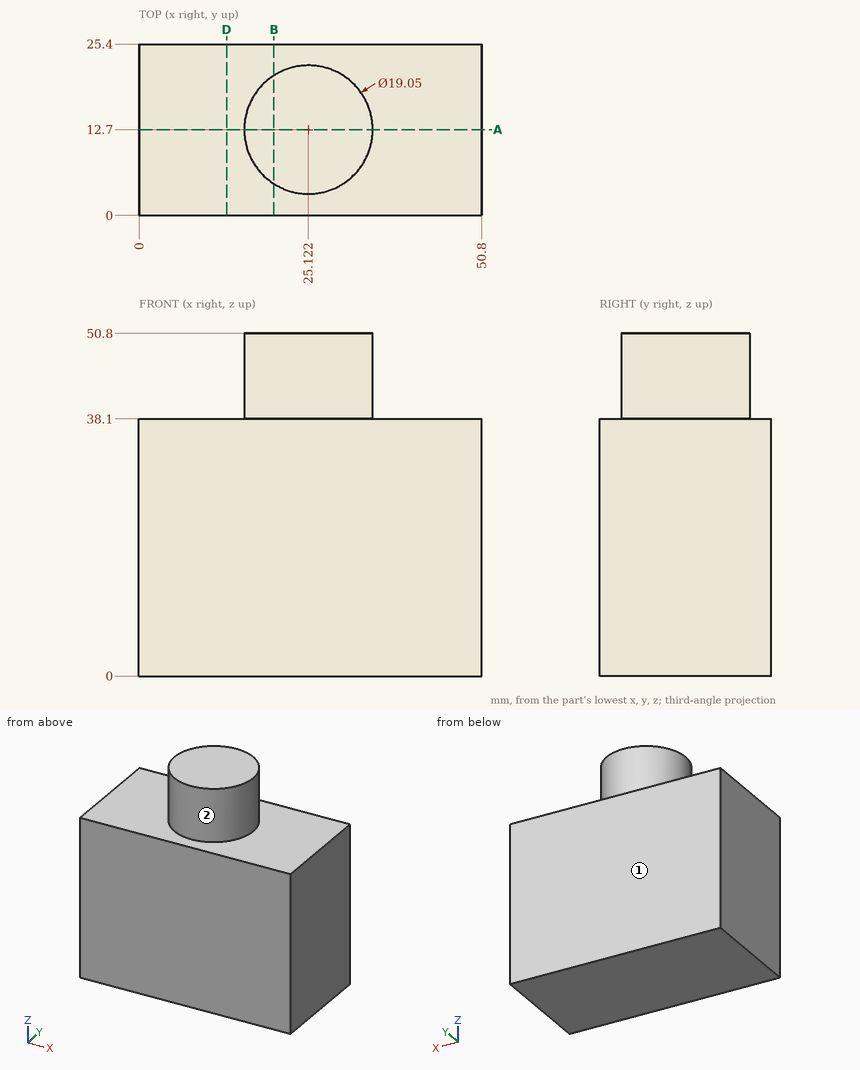
Geometry check sheet. Reference: drawing and pictorial views, mm from the part's lowest x, y, z. A direction names the side the tool comes from. Round coordinates to 2 decimals unless told otherwise and drop trailing zeros. Order: outer loops, then holes, each group sorted by start corner. A loop starts at its lowest first (then second) coordinate and runs counter-clockwise, first axis right, second up.
Q1. Cross-section at A-A, the plane y = 12.7. Enter the section's corners in (x, z), plus the area to 3 significant figures.
Filled sheet:
outline: (0, 0) - (50.8, 0) - (50.8, 38.1) - (34.65, 38.1) - (34.65, 50.8) - (15.6, 50.8) - (15.6, 38.1) - (0, 38.1) - close
area: 2,180 mm2
Q2. Scan lines: L1, parallel to Z at x = 20, y = 22.75; L2, parallel to X at y = 13.25, z = 47; L3, parallel to X at y = 16, z = 43.5. Record each from-to range of solid material in increasing order.
Filled sheet:
L1: z = 0 to 38.1
L2: x = 15.61 to 34.63
L3: x = 16.19 to 34.06
Q3. Depth check by flat-ended pin: P1, Ø5, axis at x = 33.5, z = 42.5, coming from the -Y side (1 decimal); P2, Ø10, axis at x = 41, y = 3.5, coming from the +Z side; P3, Ø6, axis at y = 6, z = 44, coming from the -X side (1 decimal). Enter the tip coordinate at first touch or a pass-through.
Filled sheet:
P1: stops at y = 5.2
P2: stops at z = 38.1
P3: stops at x = 16.3
Q4. Cross-section at D-D, the plane x = 13. Enter the section's corners in (y, z), plus the area to 3 significant figures.
Filled sheet:
outline: (0, 0) - (25.4, 0) - (25.4, 38.1) - (0, 38.1) - close
area: 968 mm2
Q5. Cross-section at B-B, the plane x = 20. Enter the section's corners in (y, z).
Filled sheet:
outline: (0, 0) - (25.4, 0) - (25.4, 38.1) - (20.73, 38.1) - (20.73, 50.8) - (4.67, 50.8) - (4.67, 38.1) - (0, 38.1) - close
Q6. Set-up check for the marked faces 1 and 2: record each of +Z, -Z, +X, -X, +Y, -Y from which the full face is reachable in a straight line by a thin tool's end or side.
Filled sheet:
face 1: +Z, -Z, +X, -X, +Y
face 2: +Z
